Model file for the job. Use its own axes, mm. Face numbers are marked on the shaded views. A direction names the side the tool comes from. Round coordinates to 2 decimals unless told otherwise and drop trailing zeros. Write each loop counter-clockwise with the first axis right and the second up, starting at its lowest first coordinate (ties: lowest second). Pieces come first, ordered by that corner, then holes. Notation, with made-up numbers: (57.25, 66.5) - (82.25, 66.5) arc R12 cw to (82.25, 82.5) - close; hole circle Ø6 at (70.25, -11). An arc over 180 degrees is marked (long way). Answer as a JSON object with one key per item and string values. Group by question number.
from build123d import *

# Parameters (mm, degrees)
SKETCH1_W          = 32.6
SKETCH1_H          = 15
SKETCH1_W_2        = 3.6
SKETCH1_H_2        = 7
SKETCH2_R          = 1.25
CUT_EXTRUDE1_DEPTH = 33.6


with BuildPart() as part:
    # Sketch1 → Revolve1 (revolve)
    with BuildSketch(Plane.XY):
        with Locations((-16.3, 7.5)):
            Rectangle(SKETCH1_W, SKETCH1_H)
        with Locations((-30.8, 18.5)):
            Rectangle(SKETCH1_W_2, SKETCH1_H_2)
        with Locations((-1.8, 18.5)):
            Rectangle(SKETCH1_W_2, SKETCH1_H_2)
    revolve(axis=Axis((0, 0, 0), (-1, 0, 0)))

    # Sketch2 → Cut-Extrude1 (cut, through all)
    with BuildSketch(Plane.ZY.offset(32.6)):
        Circle(SKETCH2_R)
    extrude(amount=-CUT_EXTRUDE1_DEPTH, mode=Mode.SUBTRACT)


solid = part.part
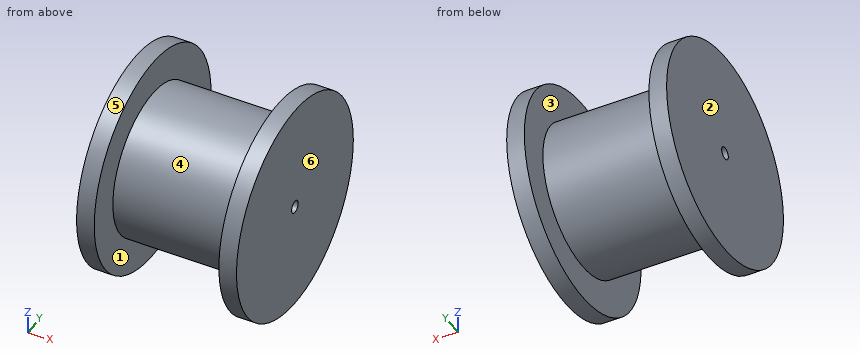
(1) Drill centre lines: line 1 (X direction, y = 13.5, z = -15); line 2 (Y direction, x = -23.5, z = 0); line 3 (Y direction, x = -17.5, z = 1). Where is each one in solid material? Low to high. Write a range as from..to.
(2) Pull direction X, two halves, no side cores. Call the marked faces 3, 4, 5 and 6: pulls with the +X half, pulls with the -X half, needs draft (parallel to the pull), parting line crosses it, or undercut.
(3) 3-axis set-ups, long thin cutter, end or side, ignore diameter. For the marked faces 1 and 2: which of +Z, -Z, +X, -X, +Y, -Y reach the whole face in a straight line?
(4) Slice it at A-A (y = 0). Write the cut outline in (x, z), then the cut area to 3 significant figures.
(5) Slice it at D-D (y = 13.5). Write the cut outline in (x, z).
(6) Slice it at C-C (x = -19). Write the cut outline in (y, z).
(7) Flat gauge pins, fed straight in: pin 1 (10 mm diameter, centred on x = -4.5, y = -15, fed in from +Z); pin 2 (8 mm diameter, centred on x = -27, z = -1.5, fed in from -Y); pin 3 (12 mm diameter, centred on x = -11, y = 16.5, fed in from +Z); pin 4 (8 mm diameter, centred on x = -5.5, y = 2, fed in from +Z). Where does each tip first touch, or does it go through?
Answer:
{
 "1": {"line 1": "-32.6..-29, -3.6..0", "line 2": "-15..-1.25, 1.25..15", "line 3": "-14.97..-0.75, 0.75..14.97"},
 "2": {"face 3": "undercut", "face 4": "undercut", "face 5": "needs draft", "face 6": "pulls with the +X half"},
 "3": {"face 1": "none", "face 2": "+Z, -Z, -X, +Y, -Y"},
 "4": {"outline": "(-32.6, -22) - (-29, -22) - (-29, -15) - (-3.6, -15) - (-3.6, -22) - (0, -22) - (0, -1.25) - (-32.6, -1.25) - close; (-32.6, 1.25) - (0, 1.25) - (0, 22) - (-3.6, 22) - (-3.6, 15) - (-29, 15) - (-29, 22) - (-32.6, 22) - close", "area": "997 mm²"},
 "5": {"outline": "(-32.6, -17.37) - (-29, -17.37) - (-29, -6.54) - (-3.6, -6.54) - (-3.6, -17.37) - (0, -17.37) - (0, 17.37) - (-3.6, 17.37) - (-3.6, 6.54) - (-29, 6.54) - (-29, 17.37) - (-32.6, 17.37) - close"},
 "6": {"outline": "circle Ø30 at (0, 0); hole circle Ø2.5 at (0, 0)"},
 "7": {"pin 1": "z = 19.55", "pin 2": "y = -22", "pin 3": "z = 10.71", "pin 4": "z = 22"}
}
